The listing builds one solid part. Answer for the finished solid, in the listing's coordinates (mm). Face numbers are marked on the shaded views. A direction names the side the tool comes from. Coordinates: 2 decimals unless noted, no trailing zeros. Order: outer loops, then holes, each group sorted by start corner. A loop starts at its lowest first (then second) coordinate and runs counter-clockwise, first axis right, second up. Notation, with made-up numbers: (35.25, -5.75) -> (60.25, -5.75) arc R30 cw to (60.25, 30.25) -> close; hole circle Ø2 at (-32.5, 85.5). An arc over 180 degrees is marked (long way). Answer in a Markdown table with one row per item.
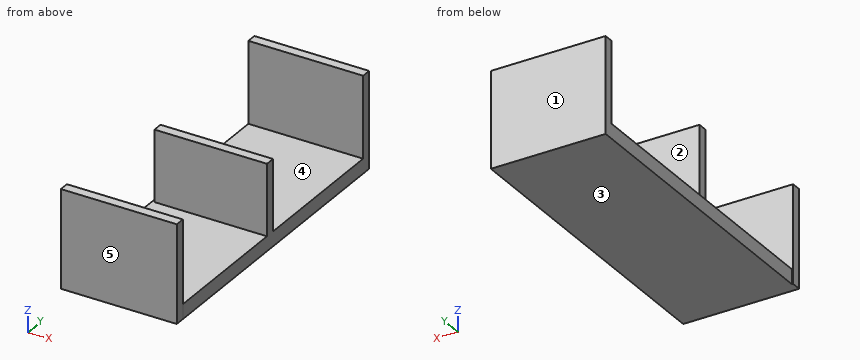
```python
from build123d import *

# Parameters (mm, degrees)
F0_W     = 59.5921203494
F0_H     = 152.5296419859
F1_DEPTH = 7.62
F3_W     = 60.1832810789
F3_H     = 50.7983006537
F4_DEPTH = 5.08
F5_W     = 58.4103576839
F5_H     = 36.9284590706
F6_DEPTH = 5.08
F7_W     = 59.5921203494
F7_H     = 49.8682297766
F8_DEPTH = 5.08


with BuildPart() as f1:
    # F0 (on Top) → F1 (new body)
    with BuildSketch(Plane.XY):
        Rectangle(F0_W, F0_H)
    extrude(amount=F1_DEPTH)

    # F3 (on offset) → F4 (join)
    with BuildSketch(Plane.XZ.offset(76.2648209929)):
        with Locations((-0.3228811547, 25.3991503268)):
            Rectangle(F3_W, F3_H)
    extrude(amount=F4_DEPTH)

    # F5 (on Front) → F6 (join)
    with BuildSketch(Plane.XZ):
        with Locations((0.5908813328, 26.0842295353)):
            Rectangle(F5_W, F5_H)
    extrude(amount=F6_DEPTH)

    # F7 (on face) → F8 (join)
    with BuildSketch(Plane(origin=(0, 76.2648209929, 0), x_dir=(-1, 0, 0), z_dir=(0, 1, 0))):
        with Locations((0, 24.9341148883)):
            Rectangle(F7_W, F7_H)
    extrude(amount=F8_DEPTH)


solid = f1.part
```
(1) A cutting plane is placed at B-B, the plane x = -5. Determine the outline of the cut face in (y, z).
Check values:
| item | result |
|---|---|
| outline | (-81.34, 0) -> (81.34, 0) -> (81.34, 49.87) -> (76.26, 49.87) -> (76.26, 7.62) -> (0, 7.62) -> (0, 44.55) -> (-5.08, 44.55) -> (-5.08, 7.62) -> (-76.26, 7.62) -> (-76.26, 50.8) -> (-81.34, 50.8) -> close |
(2) Find the intervals of material crossed by line 1 along Y through (x, z) = (8, 28.5); line 2 along Y through (x, z) = (5, 48); line 3 along Z through (x, y) = (18.5, 4.5), in increasing order. Write a range as from..to.
Check values:
| item | result |
|---|---|
| line 1 | -81.34..-76.26, -5.08..0, 76.26..81.34 |
| line 2 | -81.34..-76.26, 76.26..81.34 |
| line 3 | 0..7.62 |
(3) Flat-ended cylindrical pins translate along their axes: pin 1 (5.5 mm diameter, centred on y = -2.5, z = 24.5, fed in from -X); pin 2 (5 mm diameter, centred on x = -13, y = -17, fed in from +Z); pin 3 (1.5 mm diameter, centred on x = 11, y = -2.5, fed in from +Z). Find the tip coordinate at first contact, or state that the pin passes through.
Check values:
| item | result |
|---|---|
| pin 1 | x = -28.61 |
| pin 2 | z = 7.62 |
| pin 3 | z = 44.55 |
(4) For a pull along Y with two mould halves and no side action, classify the marked faces 3, 4 and 5 as released by +Y, released by -Y, zero draft, split by the parting line, or undercut.
Check values:
| item | result |
|---|---|
| face 3 | zero draft |
| face 4 | undercut |
| face 5 | released by -Y |
(5) A cutting plane is placed at A-A, the plane z = 35. Determine the outline of the cut face in (x, y).
Check values:
| item | result |
|---|---|
| outline | (-30.41, -81.34) -> (29.77, -81.34) -> (29.77, -76.26) -> (-30.41, -76.26) -> close; (-29.8, 76.26) -> (29.8, 76.26) -> (29.8, 81.34) -> (-29.8, 81.34) -> close; (-28.61, -5.08) -> (29.8, -5.08) -> (29.8, 0) -> (-28.61, 0) -> close |
(6) A cutting plane is placed at C-C, the plane y = 42.5. Determine the outline of the cut face in (x, z), then the cut area to 3 significant figures.
Check values:
| item | result |
|---|---|
| outline | (-29.8, 0) -> (29.8, 0) -> (29.8, 7.62) -> (-29.8, 7.62) -> close |
| area | 454 mm² |
(7) Which of the six approach directions +Z, -Z, +X, -X, +Y, -Y give full straight-line access (tool end or side, diameter ignored) to the marked faces 1 and 2?
Check values:
| item | result |
|---|---|
| face 1 | +Z, -Z, +X, -X, +Y |
| face 2 | +Z, +X, -X |
